from build123d import *

# Parameters (mm, degrees)
SKETCH1_R           = 7.62
BOSS_EXTRUDE1_DEPTH = 76.2
CUT_EXTRUDE1_DEPTH  = 51.8
CUT_EXTRUDE2_DEPTH  = 39.1
SKETCH4_R           = 10.16
CUT_EXTRUDE3_DEPTH  = 166.1
CUT_EXTRUDE4_DEPTH  = 4.445
CUT_EXTRUDE5_DEPTH  = 6.35


with BuildPart() as part:
    # Sketch1 → Boss-Extrude1 (new body, symmetric)
    with BuildSketch(Plane.XY):
        with BuildLine():
            Line((0, 0), (0, 50.8))
            Line((0, 50.8), (12.7, 50.8))
            Line((12.7, 50.8), (12.7, 135.89))
            ThreePointArc((12.7, 135.89), (11.584076836, 138.584076836), (8.89, 139.7))
            Line((8.89, 139.7), (0, 139.7))
            Line((0, 139.7), (0, 165.1))
            Line((0, 165.1), (12.7, 165.1))
            Line((12.7, 165.1), (38.1, 139.7))
            Line((38.1, 139.7), (38.1, 50.8))
            Line((38.1, 50.8), (50.8, 50.8))
            Line((50.8, 50.8), (50.8, 38.1))
            Line((50.8, 38.1), (203.2, 38.1))
            Line((203.2, 38.1), (203.2, 31.75))
            Line((203.2, 31.75), (196.85, 31.75))
            Line((196.85, 31.75), (190.5, 12.7))
            Line((190.5, 12.7), (196.85, -6.35))
            Line((196.85, -6.35), (203.2, -6.35))
            Line((203.2, -6.35), (203.2, -12.7))
            Line((203.2, -12.7), (95.25, -12.7))
            Line((95.25, -12.7), (95.25, 12.7))
            Line((95.25, 12.7), (50.8, 12.7))
            Line((50.8, 12.7), (50.8, 0))
            Line((50.8, 0), (0, 0))
        make_face()
        with Locations((25.4, 41.275)):
            Circle(SKETCH1_R, mode=Mode.SUBTRACT)
        Polygon((146.408669031, 8.298741154), (138.995217137, 31.115), (115.004782863, 31.115), (107.591330969, 8.298741154), (127, -5.802482309), align=None, mode=Mode.SUBTRACT)
    extrude(amount=BOSS_EXTRUDE1_DEPTH, both=True)

    # Sketch2 → Cut-Extrude1 (cut, through all)
    with BuildSketch(Plane(origin=(0, 38.1, 0), x_dir=(1, 0, 0), z_dir=(0, 1, 0))):
        with BuildLine():
            Line((57.15, 59.69), (57.15, 12.310112434))
            ThreePointArc((57.15, 12.310112434), (60.162452878, 6.907957382), (66.341584002, 6.631388955))
            Line((66.341584002, 6.631388955), (120.316584002, 33.640011057))
            ThreePointArc((120.316584002, 33.640011057), (122.877155052, 35.981187414), (123.825, 39.318734537))
            Line((123.825, 39.318734537), (123.825, 59.69))
            ThreePointArc((123.825, 59.69), (121.965128061, 64.180128061), (117.475, 66.04))
            Line((117.475, 66.04), (63.5, 66.04))
            ThreePointArc((63.5, 66.04), (59.009871939, 64.180128061), (57.15, 59.69))
        make_face()
        with BuildLine():
            Line((78.20049599, 4.862340879), (147.285148797, 39.431702264))
            ThreePointArc((147.285148797, 39.431702264), (160.392932197, 37.380552912), (162.731634589, 24.321009641))
            Line((162.731634589, 24.321009641), (129.688781962, -45.506634528))
            ThreePointArc((129.688781962, -45.506634528), (68.606892677, -56.445176375), (78.20049599, 4.862340879))
        make_face()
        with BuildLine():
            Line((131.290134658, -58.243894245), (161.338708783, 5.256105755))
            ThreePointArc((161.338708783, 5.256105755), (163.681799397, 7.905154776), (167.078505776, 8.89))
            Line((167.078505776, 8.89), (177.8, 8.89))
            ThreePointArc((177.8, 8.89), (182.290128061, 7.030128061), (184.15, 2.54))
            Line((184.15, 2.54), (184.15, -60.96))
            ThreePointArc((184.15, -60.96), (182.290128061, -65.450128061), (177.8, -67.31))
            Line((177.8, -67.31), (137.029931652, -67.31))
            ThreePointArc((137.029931652, -67.31), (131.664776876, -64.35670638), (131.290134658, -58.243894245))
        make_face()
        with BuildLine():
            ThreePointArc((188.57162547, 22.277294118), (174.627718402, 58.576263546), (135.906341971, 62.140352941))
            ThreePointArc((135.906341971, 62.140352941), (131.513776952, 48.932212079), (144.721917814, 44.539647059))
            ThreePointArc((144.721917814, 44.539647059), (162.747386153, 42.880501996), (169.238515305, 25.982705882))
            ThreePointArc((169.238515305, 25.982705882), (177.052364505, 14.463444917), (188.57162547, 22.277294118))
        make_face()
    extrude(amount=-CUT_EXTRUDE1_DEPTH, mode=Mode.SUBTRACT)

    # Sketch3 → Cut-Extrude2 (cut, through all)
    with BuildSketch(Plane(origin=(38.1, 0, 0), x_dir=(0, 0, -1), z_dir=(1, 0, 0))):
        Polygon((-40.64, 133.35), (40.64, 133.35), (57.15, 116.84), (57.15, 73.66), (40.64, 57.15), (-40.64, 57.15), (-57.15, 73.66), (-57.15, 116.84), align=None)
    extrude(amount=-CUT_EXTRUDE2_DEPTH, mode=Mode.SUBTRACT)

    # Sketch4 → Cut-Extrude3 (cut, through all)
    with BuildSketch(Plane.XZ):
        with Locations((25.4, 15.875)):
            Circle(SKETCH4_R)
        with Locations((25.4, -15.875)):
            Circle(SKETCH4_R)
    extrude(amount=-CUT_EXTRUDE3_DEPTH, mode=Mode.SUBTRACT)

    # Sketch6 → Cut-Extrude4 (cut)
    with BuildSketch(Plane.XZ):
        Polygon((25.4, 0.762), (36.086504784, 5.188495216), (40.513, 15.875), (36.086504784, 26.561504784), (25.4, 30.988), (14.713495216, 26.561504784), (10.287, 15.875), (14.713495216, 5.188495216), align=None)
        Polygon((25.4, -30.988), (36.086504784, -26.561504784), (40.513, -15.875), (36.086504784, -5.188495216), (25.4, -0.762), (14.713495216, -5.188495216), (10.287, -15.875), (14.713495216, -26.561504784), align=None)
    extrude(amount=-CUT_EXTRUDE4_DEPTH, mode=Mode.SUBTRACT)

    # Sketch7 → Cut-Extrude5 (cut)
    with BuildSketch(Plane.XY.offset(76.2)):
        Polygon((40.064696837, 41.275), (32.732348419, 53.975), (18.067651581, 53.975), (10.735303163, 41.275), (18.067651581, 28.575), (32.732348419, 28.575), align=None)
    cut_extrude5 = extrude(amount=-CUT_EXTRUDE5_DEPTH, mode=Mode.SUBTRACT)

    # Mirror1: Cut-Extrude5 across plane
    add(cut_extrude5.mirror(Plane.XY), mode=Mode.SUBTRACT)


solid = part.part
CAD build for the part. Positions are in the model's coordinates, mm. A direction names the side the tool comes from. Coordinates: 2 decimals unless noted, no trailing zeros. Write each loop counter-clockwise with the first axis right and the second up, starting at its lowest first coordinate (ties: lowest second). Pieces come first, ordered by that corner, then holes. Notation, with made-up numbers: M 10.5,-11.75 L 47.5,-11.75 A22 cw 47.5,3.25 Z; hole C 78.5,-25.75 d7. An arc over 180 degrees is marked long. Answer as a JSON object with one key per item and string values. Group by question number.
1) Saw through at D-D (z = -53.34). Give the number of separate pieces and of enclosed holes in the cut face, plus the area to 3 significant figures.
2) Mould opens along X. For faces 1 (the face through (26, 95, 57.15)), 2 (the face through (38.1, 135, 1)), 3 (the face through (131.71, 34.66, 64.43)) say: +X half, -X half, draft (parallel to the pull), parting line (faces both ways), or undercut.
3) Saw through at B-B (x = 87). Write the cut outline in (y, z), plus the area to 3 significant figures.
4) Wall check: line 1 (Z direction, x = 25, y = 149); line 2 (Z direction, x = 179, y = 36.5); line 3 (Y direction, x = 57, z = -24). Give the ranges that are in metal, low to high. Write a range as from..to.
5) Saw through at A-A (y = 61). Write the cut outline in (x, z), plus the area to 3 significant figures.
6) Pin check, flat tips, straight feed: pin 1 Ø4 at (y, z) = (5, 39) entering from +X; pin 2 Ø5 at (x, z) = (24, 74) entering from +Y; pin 3 Ø16.5 at (x, z) = (25.4, -15.875) entering from -Y; pin 4 Ø23.5 at (x, z) = (25.4, 15.875) entering from +Y. Stop position of each tip, or through.
7) Tool access for faces 4 (the face through (32, 47, 69.85)), 5 (the face through (172, 13, -8.89)), 6 (the face through (111.35, 19.87, -25.2)): list every direction of +Z, -Z, +X, -X, +Y, -Y with a clear straight run to the whole face (end or side of a thin tool).
8) Saw through at C-C (y = 99). Write the cut outline in (x, z), plus the area to 3 significant figures.
Values follow:
{
 "1": {"separate pieces": "5", "enclosed holes": "1", "area": "5,080 mm2"},
 "2": {"face 1": "draft", "face 2": "+X half", "face 3": "undercut"},
 "3": {"outline": "M 12.7,-76.2 L 38.1,-76.2 L 38.1,-66.04 L 12.7,-66.04 Z; M 12.7,-16.97 L 38.1,-16.97 L 38.1,-9.27 L 12.7,-9.27 Z; M 12.7,66.41 L 38.1,66.41 L 38.1,76.2 L 12.7,76.2 Z", "area": "702 mm2"},
 "4": {"line 1": "z = -76.2..-26.03, -5.72..5.72, 26.03..76.2", "line 2": "z = -76.2..-54.68, -14.29..-8.78, 67.2..76.2", "line 3": "y = 12.7..38.1"},
 "5": {"outline": "M 12.7,-76.2 L 38.1,-76.2 L 38.1,-44.49 L 12.7,-44.49 Z; M 12.7,44.49 L 38.1,44.49 L 38.1,76.2 L 12.7,76.2 Z", "area": "1,610 mm2"},
 "6": {"pin 1": "stops at x = 193.73", "pin 2": "stops at y = 156.3", "pin 3": "passes through", "pin 4": "stops at y = 164.15"},
 "7": {"face 4": "+Z", "face 5": "+Y, -Y", "face 6": "+Z, -Z"},
 "8": {"outline": "M 12.7,-76.2 L 38.1,-76.2 L 38.1,-57.15 L 12.7,-57.15 Z; M 12.7,57.15 L 38.1,57.15 L 38.1,76.2 L 12.7,76.2 Z", "area": "968 mm2"}
}
